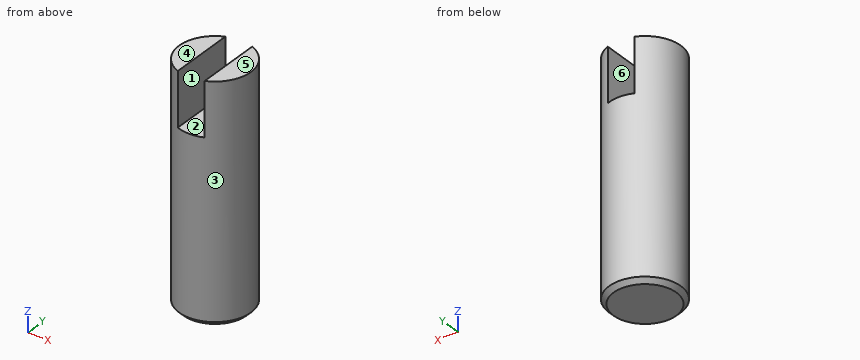
Autodesk Inventor part; units mm, degrees
ref_plane "YZ Plane" through (0, 0, 0) normal (1, 0, 0) x (0, 1, 0)
ref_plane "XZ Plane" through (0, 0, 0) normal (0, 1, 0) x (-1, 0, 0)
ref_plane "XY Plane" through (0, 0, 0) normal (0, 0, 1) x (1, 0, 0)
sketch "草图1" plane through (0, 0, 0) normal (0, 0, 1) x (1, 0, 0)
  circle A0 centre (0, 0) radius 2
  dimension "d0" = 4
extrude "拉伸1" add sketch "草图1" along normal blind 13
sketch "草图2" plane through (0, 0, 13) normal (0, 0, 1) x (1, 0, 0)
  line L0 (-0.75, 2) -> (0.75, 2)
  line L1 (0.75, 2) -> (0.75, -2)
  line L2 (0.75, -2) -> (-0.75, -2)
  line L3 (-0.75, -2) -> (-0.75, 2)
  line L4 (0, 0) -> (0, 2)
  circle A0 centre (0, 0) radius 2
  dimension "d3" = 1.5
extrude "拉伸2" cut sketch "草图2" against normal blind 3 contours L0 A0 L3 | L0 L1 A0 | A0 L1 L3 | A0 L2 L3 | L1 L2 A0
thread "螺纹1"
chamfer "倒角1" distance 0.25 angle 45 1 edges at (-2, 0, 0)
properties part number "砂轮电机皮带轮固定螺丝"
The model under review builds one solid part; all positions refer to its coordinate system, in mm. Face numbers are marked on the shaded views. A direction names the side the tool comes from. Coordinates: 2 decimals unless noted, no trailing zeros. Order: outer loops, then holes, each group sorted by start corner. A loop starts at its lowest first (then second) coordinate and runs counter-clockwise, first axis right, second up. Notation, with made-up numbers: (-22, 30.5) -> (8, 30.5) arc R19 cw to (8, 44.5) -> close; hole circle Ø10 at (88.25, 84). An arc over 180 degrees is marked (long way). Answer in a Markdown table with one row per item.
(1) The part is to be moulded in two halves that separate along X. For the marked faces 1, 2, 3 and 4, say which applies: +X half, -X half, draft (parallel to the pull), parting line (faces both ways), or undercut.
Answers:
| item | result |
|---|---|
| face 1 | undercut |
| face 2 | undercut |
| face 3 | parting line |
| face 4 | draft |
(2) Consider section A-A (y = 0). Write out the cut boundary in (x, z).
Answers:
| item | result |
|---|---|
| outline | (-2, 0.25) -> (-1.75, 0) -> (1.75, 0) -> (2, 0.25) -> (2, 13) -> (0.75, 13) -> (0.75, 10) -> (-0.75, 10) -> (-0.75, 13) -> (-2, 13) -> close |
(3) Consider section B-B (z = 7.25). Write out the cut boundary in (x, y).
Answers:
| item | result |
|---|---|
| outline | circle Ø4 at (0, 0) |
(4) Consider section C-C (x = 0). Write out the cut boundary in (y, z).
Answers:
| item | result |
|---|---|
| outline | (-2, 0.25) -> (-1.75, 0) -> (1.75, 0) -> (2, 0.25) -> (2, 10) -> (-2, 10) -> close |
(5) Wall thickness on line 1 along X through (y, z) = (-1.2, 11.25); line 2 along Z through (x, y) = (-0.55, -0.8); line 3 along Y through (x, z) = (-1.35, 2.5): over which ranges is each line inside the solid? List them lowest first.
Answers:
| item | result |
|---|---|
| line 1 | -1.6 to -0.75, 0.75 to 1.6 |
| line 2 | 0 to 10 |
| line 3 | -1.48 to 1.48 |
(6) Consider section D-D (z = 11.5). Write out the cut boundary in (x, y), plus the area to 3 significant figures.
Answers:
| item | result |
|---|---|
| outline | (-0.75, -1.85) -> (-0.75, 1.85) arc R2 ccw to start; (0.75, -1.85) arc R2 ccw to (0.75, 1.85) -> close |
| area | 6.71 mm² |
(7) Insertion check: pin 1 (0.8 mm diameter, centred on x = 0, y = -0.5, fed in from +Z). The pin has a flat end and moves straight along its axis. Give the tip position at first contact, or say it passes through.
Answers:
| item | result |
|---|---|
| pin 1 | z = 10 |
(8) Machinability: for the marked faces 5 and 6, which of the approach directions +Z, -Z, +X, -X, +Y, -Y give a long, thin tool a straight path to every point of the face, cutting with its end or side? Answer none if there is none.
Answers:
| item | result |
|---|---|
| face 5 | +Z, +X, -X, +Y, -Y |
| face 6 | +Z, +Y, -Y |
